Answer from the drawing. Dimensions are ordinates in mm from the lowest x, y and z of the part. Give positions to 0.01 mm unless a question says otherwise; leave off trailing zeros. Loops run counter-clockwise (first coordinate to the right, second up) from the corner with the lowest first, then second, coordinate; pieces in that order, holes last. Notation, with made-up numbers: (0.25, 57.5) - (56.25, 57.5) arc R11 ccw to (56.25, 67.5) - close; hole circle Ø11 at (22, 65). An arc over 180 degrees is marked (long way). One line per item, written item: value.
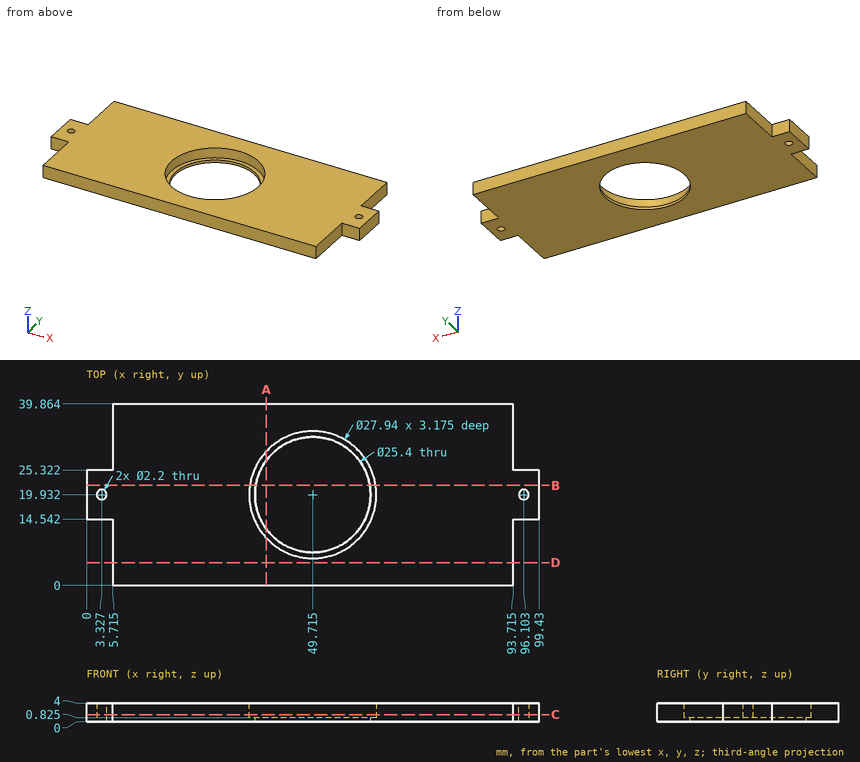
1. Flat-ended cylindrical pins translate along their axes: pin 1 Ø2 at (x, z) = (3, 2) entering from -Y; pin 2 Ø2 at (x, z) = (97, 2.5) entering from +Y. Find the tip coordinate at first contact, or state that the pin passes through.
Output:
pin 1: stops at y = 14.54
pin 2: stops at y = 25.32
2. Section C-C (z = 1.55) is taken. Write down the section's boundary in (x, y) (1 decimal), and give its area (3 significant figures).
Output:
outline: (0, 14.5) - (5.7, 14.5) - (5.7, 0) - (93.7, 0) - (93.7, 14.5) - (99.4, 14.5) - (99.4, 25.3) - (93.7, 25.3) - (93.7, 39.9) - (5.7, 39.9) - (5.7, 25.3) - (0, 25.3) - close; hole circle Ø2.2 at (3.3, 19.9); hole circle Ø27.9 at (49.7, 19.9); hole circle Ø2.2 at (96.1, 19.9)
area: 3,010 mm²
3. Section B-B (y = 22) is taken. Write down the section's boundary in (x, z) (1 decimal), and give its area (3 significant figures).
Output:
outline: (0, 0) - (37.2, 0) - (37.2, 0.8) - (35.9, 0.8) - (35.9, 4) - (0, 4) - close; (62.2, 0) - (99.4, 0) - (99.4, 4) - (63.5, 4) - (63.5, 0.8) - (62.2, 0.8) - close
area: 289 mm²
4. Section D-D (y = 5) is taken. Write down the section's boundary in (x, z) (1 decimal), and give its area (3 significant figures).
Output:
outline: (5.7, 0) - (93.7, 0) - (93.7, 4) - (5.7, 4) - close
area: 352 mm²
5. Find the intervals of material crossed by line 1 along X through (y, z) = (10.5, 1.55) (1 decimal); line 2 along X through (y, z) = (22, 2); line 3 along X through (y, z) = (4.5, 0.65) (1 decimal), in increasing order.
Output:
line 1: x = 5.7 to 39.4, 60 to 93.7
line 2: x = 0 to 35.9, 63.53 to 99.43
line 3: x = 5.7 to 93.7
6. Section A-A (x = 39.5) is taken. Write down the section's boundary in (y, z) (1 decimal).
Output:
outline: (0, 0) - (12.4, 0) - (12.4, 0.8) - (10.4, 0.8) - (10.4, 4) - (0, 4) - close; (27.5, 0) - (39.9, 0) - (39.9, 4) - (29.5, 4) - (29.5, 0.8) - (27.5, 0.8) - close
